```python
from build123d import *

# Parameters (mm, degrees)
SKETCH1_W            = 50.8
SKETCH1_H            = 38.1
SKETCH1_R            = 13.335
BOSS_EXTRUDE2_DEPTH  = 25.4
CUT_EXTRUDE1_REACH   = 42.66
SKETCH2_W            = 25.4
SKETCH2_H            = 2.54
SKETCH3_R            = 2.665
CUT_EXTRUDE2_DEPTH   = 53.363441445
CUT_EXTRUDE3_DEPTH   = 10
CUT_EXTRUDE4_START   = -1.5
CUT_EXTRUDE4_DEPTH   = 1.5
SKETCH6_W            = 50.8
SKETCH6_H            = 38.1
SKETCH6_R            = 6.477
BOSS_EXTRUDE3_DEPTH  = 6.35
BOSS_EXTRUDE4_DEPTH  = 44.45
BOSS_EXTRUDE5_DEPTH  = 6.604
SKETCH11_W           = 57.15
SKETCH11_H           = 127
BOSS_EXTRUDE6_DEPTH  = 10.16
CUT_EXTRUDE6_REACH   = 147.3
SKETCH12_R           = 7.62
SKETCH13_R           = 14.351
CUT_EXTRUDE7_DEPTH   = 7.9375
CUT_EXTRUDE8_REACH   = 147.3
CUT_EXTRUDE11_REACH  = 141.019
CUT_EXTRUDE12_REACH  = 147.3
SKETCH16_W           = 57.15
SKETCH16_H           = 7.545
SKETCH17_W           = 17.78
SKETCH17_H           = 23.9
BOSS_EXTRUDE7_DEPTH  = 3.175
BOSS_EXTRUDE8_DEPTH  = 3.175
BOSS_EXTRUDE10_DEPTH = 3.175
SKETCH20_W           = 17.78
SKETCH20_H           = 23.9
BOSS_EXTRUDE11_DEPTH = 3.175
CUT_EXTRUDE13_REACH  = 129.55
SKETCH21_R           = 2.665


with BuildPart() as part:
    # Sketch1 → Boss-Extrude2 (new body)
    with BuildSketch(Plane(origin=(0, 0, 0), x_dir=(1, 0, 0), z_dir=(0, 1, 0))):
        Rectangle(SKETCH1_W, SKETCH1_H)
        with Locations(Location((0, 0, 0), (0, 0, 270))):
            Circle(SKETCH1_R, mode=Mode.SUBTRACT)
    extrude(amount=BOSS_EXTRUDE2_DEPTH)

    # Sketch2 → Cut-Extrude1 (cut, up to next)
    with BuildSketch(Plane(origin=(0, 25.4, 0), x_dir=(1, 0, 0), z_dir=(0, 1, 0)), mode=Mode.PRIVATE) as cut_extrude1_sk1:
        with Locations((12.7, 0)):
            Rectangle(SKETCH2_W, SKETCH2_H)
    cut_extrude1_tool1 = extrude(cut_extrude1_sk1.sketch, amount=-CUT_EXTRUDE1_REACH, mode=Mode.PRIVATE) & part.part
    add(cut_extrude1_tool1.solids().sort_by_distance((12.7, 25.4, 0))[0], mode=Mode.SUBTRACT)

    # Sketch3 → Cut-Extrude2 (cut, through all)
    with BuildSketch(Plane.XY.offset(19.05)):
        with Locations((19.05, 19.05)):
            Circle(SKETCH3_R)
        with Locations((19.05, 6.35)):
            Circle(SKETCH3_R)
    extrude(amount=-CUT_EXTRUDE2_DEPTH, mode=Mode.SUBTRACT)

    # Sketch4 → Cut-Extrude3 (cut)
    with BuildSketch(Plane(origin=(0, 0, -19.05), x_dir=(-1, 0, 0), z_dir=(0, 0, -1))):
        Polygon((-19.05, 24.823502692), (-24.05, 21.936751346), (-24.05, 16.163248654), (-19.05, 13.276497308), (-14.05, 16.163248654), (-14.05, 21.936751346), align=None)
        Polygon((-19.05, 12.123502692), (-24.05, 9.236751346), (-24.05, 3.463248654), (-19.05, 0.576497308), (-14.05, 3.463248654), (-14.05, 9.236751346), align=None)
    extrude(amount=-CUT_EXTRUDE3_DEPTH, mode=Mode.SUBTRACT)

    # Sketch5 → Cut-Extrude4 (cut)
    with BuildSketch(Plane(origin=(0, 25.4, 0), x_dir=(1, 0, 0), z_dir=(0, 1, 0)).offset(CUT_EXTRUDE4_START)):
        with BuildLine():
            Line((-19.05, -19.05), (-9.429268927, -9.429268927))
            ThreePointArc((-9.429268927, -9.429268927), (4.509949975, -12.549206199), (13.27438605, -1.27))
            Line((13.27438605, -1.27), (25.4, -1.27))
            Line((25.4, -1.27), (25.4, -19.05))
            Line((25.4, -19.05), (-19.05, -19.05))
        make_face()
    extrude(amount=CUT_EXTRUDE4_DEPTH, mode=Mode.SUBTRACT)

    # Sketch6 → Boss-Extrude3 (add)
    with BuildSketch(Plane(origin=(0, 25.4, 0), x_dir=(1, 0, 0), z_dir=(0, 1, 0))):
        Rectangle(SKETCH6_W, SKETCH6_H)
        with Locations(Location((0, 0, 0), (0, 0, 270))):
            Circle(SKETCH6_R, mode=Mode.SUBTRACT)
    extrude(amount=BOSS_EXTRUDE3_DEPTH)

    # Sketch8 → Boss-Extrude4 (add)
    with BuildSketch(Plane(origin=(0, 31.75, 0), x_dir=(1, 0, 0), z_dir=(0, 1, 0))):
        with BuildLine():
            Line((-25.4, 19.05), (25.4, 19.05))
            Line((25.4, 19.05), (25.4, 0))
            Line((25.4, 0), (6.477, 0))
            ThreePointArc((6.477, 0), (0, 6.477), (-6.477, 0))
            Line((-6.477, 0), (-25.4, 0))
            Line((-25.4, 0), (-25.4, 19.05))
        make_face()
    extrude(amount=BOSS_EXTRUDE4_DEPTH)

    # Sketch10 → Boss-Extrude5 (add)
    with BuildSketch(Plane(origin=(0, 76.2, 0), x_dir=(1, 0, 0), z_dir=(0, 1, 0))):
        with BuildLine():
            Line((-25.4, 19.05), (-25.4, 0))
            Line((-25.4, 0), (-13.97, 0))
            ThreePointArc((-13.97, 0), (0, 13.97), (13.97, 0))
            Line((13.97, 0), (25.4, 0))
            Line((25.4, 0), (25.4, 19.05))
            Line((25.4, 19.05), (-25.4, 19.05))
        make_face()
    extrude(amount=BOSS_EXTRUDE5_DEPTH)

    # Sketch11 → Boss-Extrude6 (add)
    with BuildSketch(Plane(origin=(0, 82.804, 0), x_dir=(1, 0, 0), z_dir=(0, 1, 0))):
        with Locations((0, 44.45)):
            Rectangle(SKETCH11_W, SKETCH11_H)
    extrude(amount=BOSS_EXTRUDE6_DEPTH)

    # Sketch12 → Cut-Extrude6 (cut, up to next)
    with BuildSketch(Plane(origin=(0, 92.964, 0), x_dir=(1, 0, 0), z_dir=(0, 1, 0)), mode=Mode.PRIVATE) as cut_extrude6_sk1:
        with Locations(Location((0, 0, 0), (0, 0, 270))):
            Circle(SKETCH12_R)
    cut_extrude6_tool1 = extrude(cut_extrude6_sk1.sketch, amount=-CUT_EXTRUDE6_REACH, mode=Mode.PRIVATE) & part.part
    add(cut_extrude6_tool1.solids().sort_by_distance((0, 92.964, 0))[0], mode=Mode.SUBTRACT)

    # Sketch13 → Cut-Extrude7 (cut)
    with BuildSketch(Plane(origin=(0, 92.964, 0), x_dir=(1, 0, 0), z_dir=(0, 1, 0))):
        with Locations(Location((0, 0, 0), (0, 0, 270))):
            Circle(SKETCH13_R)
    extrude(amount=-CUT_EXTRUDE7_DEPTH, mode=Mode.SUBTRACT)

    # Sketch14 → Cut-Extrude8 (cut, up to next)
    with BuildSketch(Plane(origin=(0, 92.964, 0), x_dir=(1, 0, 0), z_dir=(0, 1, 0)), mode=Mode.PRIVATE) as cut_extrude8_sk1:
        with BuildLine():
            Line((-19.177, 65.405), (-19.177, 71.755))
            ThreePointArc((-19.177, 71.755), (0, 90.932), (19.177, 71.755))
            Line((19.177, 71.755), (19.177, 65.405))
            ThreePointArc((19.177, 65.405), (0, 46.228), (-19.177, 65.405))
        make_face()
    cut_extrude8_tool1 = extrude(cut_extrude8_sk1.sketch, amount=-CUT_EXTRUDE8_REACH, mode=Mode.PRIVATE) & part.part
    add(cut_extrude8_tool1.solids().sort_by_distance((0, 92.964, -68.58))[0], mode=Mode.SUBTRACT)

    # Sketch15 → Cut-Extrude11 (cut, up to next)
    with BuildSketch(Plane.XZ.offset(-82.804), mode=Mode.PRIVATE) as cut_extrude11_sk1:
        with BuildLine():
            Line((-21.03, -88.975), (-21.03, -95.325))
            ThreePointArc((-21.03, -95.325), (-23.57, -97.865), (-26.11, -95.325))
            Line((-26.11, -95.325), (-26.11, -88.975))
            ThreePointArc((-26.11, -88.975), (-23.57, -86.435), (-21.03, -88.975))
        make_face()
    cut_extrude11_tool1 = extrude(cut_extrude11_sk1.sketch, amount=-CUT_EXTRUDE11_REACH, mode=Mode.PRIVATE) & part.part
    # Sketch15 → Cut-Extrude11 (cut, up to next)
    with BuildSketch(Plane.XZ.offset(-82.804), mode=Mode.PRIVATE) as cut_extrude11_sk2:
        with BuildLine():
            Line((26.11, -88.975), (26.11, -95.325))
            ThreePointArc((26.11, -95.325), (23.57, -97.865), (21.03, -95.325))
            Line((21.03, -95.325), (21.03, -88.975))
            ThreePointArc((21.03, -88.975), (23.57, -86.435), (26.11, -88.975))
        make_face()
    cut_extrude11_tool2 = extrude(cut_extrude11_sk2.sketch, amount=-CUT_EXTRUDE11_REACH, mode=Mode.PRIVATE) & part.part
    # Sketch15 → Cut-Extrude11 (cut, up to next)
    with BuildSketch(Plane.XZ.offset(-82.804), mode=Mode.PRIVATE) as cut_extrude11_sk3:
        with BuildLine():
            Line((26.11, -41.835), (26.11, -48.185))
            ThreePointArc((26.11, -48.185), (23.57, -50.725), (21.03, -48.185))
            Line((21.03, -48.185), (21.03, -41.835))
            ThreePointArc((21.03, -41.835), (23.57, -39.295), (26.11, -41.835))
        make_face()
    cut_extrude11_tool3 = extrude(cut_extrude11_sk3.sketch, amount=-CUT_EXTRUDE11_REACH, mode=Mode.PRIVATE) & part.part
    # Sketch15 → Cut-Extrude11 (cut, up to next)
    with BuildSketch(Plane.XZ.offset(-82.804), mode=Mode.PRIVATE) as cut_extrude11_sk4:
        with BuildLine():
            Line((-21.03, -41.835), (-21.03, -48.185))
            ThreePointArc((-21.03, -48.185), (-23.57, -50.725), (-26.11, -48.185))
            Line((-26.11, -48.185), (-26.11, -41.835))
            ThreePointArc((-26.11, -41.835), (-23.57, -39.295), (-21.03, -41.835))
        make_face()
    cut_extrude11_tool4 = extrude(cut_extrude11_sk4.sketch, amount=-CUT_EXTRUDE11_REACH, mode=Mode.PRIVATE) & part.part
    add(cut_extrude11_tool1.solids().sort_by_distance((-23.57, 82.804, -92.15))[0], mode=Mode.SUBTRACT)
    add(cut_extrude11_tool2.solids().sort_by_distance((23.57, 82.804, -92.15))[0], mode=Mode.SUBTRACT)
    add(cut_extrude11_tool3.solids().sort_by_distance((23.57, 82.804, -45.01))[0], mode=Mode.SUBTRACT)
    add(cut_extrude11_tool4.solids().sort_by_distance((-23.57, 82.804, -45.01))[0], mode=Mode.SUBTRACT)

    # Sketch16 → Cut-Extrude12 (cut, up to next)
    with BuildSketch(Plane(origin=(0, 92.964, 0), x_dir=(1, 0, 0), z_dir=(0, 1, 0)), mode=Mode.PRIVATE) as cut_extrude12_sk1:
        with Locations((0, 104.1775)):
            Rectangle(SKETCH16_W, SKETCH16_H)
    cut_extrude12_tool1 = extrude(cut_extrude12_sk1.sketch, amount=-CUT_EXTRUDE12_REACH, mode=Mode.PRIVATE) & part.part
    add(cut_extrude12_tool1.solids().sort_by_distance((0, 92.964, -104.1775))[0], mode=Mode.SUBTRACT)

    # Sketch17 → Boss-Extrude7 (add)
    with BuildSketch(Plane(origin=(25.4, 0, 0), x_dir=(0, 0, -1), z_dir=(1, 0, 0))):
        with Locations((-10.16, 11.95)):
            Rectangle(SKETCH17_W, SKETCH17_H)
        Polygon((19.05, 0), (19.05, 82.804), (0, 82.804), (0, 31.75), (-19.05, 31.75), (-19.05, 25.4), (1.27, 25.4), (1.27, 0), align=None)
    extrude(amount=BOSS_EXTRUDE7_DEPTH)

    # Sketch18 → Boss-Extrude8 (add)
    with BuildSketch(Plane.ZY.offset(25.4)):
        Polygon((-19.05, 0), (19.05, 0), (19.05, 31.75), (0, 31.75), (0, 82.804), (-19.05, 82.804), align=None)
    extrude(amount=BOSS_EXTRUDE8_DEPTH)

    # Sketch19 → Boss-Extrude10 (add)
    with BuildSketch(Plane.ZY.offset(28.575)):
        Polygon((0, 92.964), (-100.405, 92.964), (-100.405, 82.804), (-19.05, 82.804), (-19.05, 31.75), (0, 31.75), (0, 82.804), (19.05, 82.804), (19.05, 92.964), align=None)
        Polygon((0, 31.75), (-19.05, 31.75), (-19.05, 0), (19.05, 0), (19.05, 31.75), align=None)
        Polygon((-19.05, 82.804), (-100.405, 82.804), (-19.05, 31.75), align=None)
    extrude(amount=BOSS_EXTRUDE10_DEPTH)

    # Sketch20 → Boss-Extrude11 (add)
    with BuildSketch(Plane(origin=(28.575, 0, 0), x_dir=(0, 0, -1), z_dir=(1, 0, 0))):
        Polygon((19.05, 31.75), (100.405, 82.804), (100.405, 92.964), (-19.05, 92.964), (-19.05, 82.804), (0, 82.804), (0, 31.75), (-19.05, 31.75), (-19.05, 25.4), (1.27, 25.4), (1.27, 0), (19.05, 0), align=None)
        with Locations((-10.16, 11.95)):
            Rectangle(SKETCH20_W, SKETCH20_H)
    extrude(amount=BOSS_EXTRUDE11_DEPTH)

    # Sketch21 → Cut-Extrude13 (cut, up to next)
    with BuildSketch(Plane(origin=(0, 0, -19.05), x_dir=(-1, 0, 0), z_dir=(0, 0, -1)), mode=Mode.PRIVATE) as cut_extrude13_sk1:
        with Locations((22.575, 57.15)):
            Circle(SKETCH21_R)
    cut_extrude13_tool1 = extrude(cut_extrude13_sk1.sketch, amount=-CUT_EXTRUDE13_REACH, mode=Mode.PRIVATE) & part.part
    # Sketch21 → Cut-Extrude13 (cut, up to next)
    with BuildSketch(Plane(origin=(0, 0, -19.05), x_dir=(-1, 0, 0), z_dir=(0, 0, -1)), mode=Mode.PRIVATE) as cut_extrude13_sk2:
        with Locations((-22.575, 57.15)):
            Circle(SKETCH21_R)
    cut_extrude13_tool2 = extrude(cut_extrude13_sk2.sketch, amount=-CUT_EXTRUDE13_REACH, mode=Mode.PRIVATE) & part.part
    add(cut_extrude13_tool1.solids().sort_by_distance((-22.575, 57.15, -19.05))[0], mode=Mode.SUBTRACT)
    add(cut_extrude13_tool2.solids().sort_by_distance((22.575, 57.15, -19.05))[0], mode=Mode.SUBTRACT)


solid = part.part
```
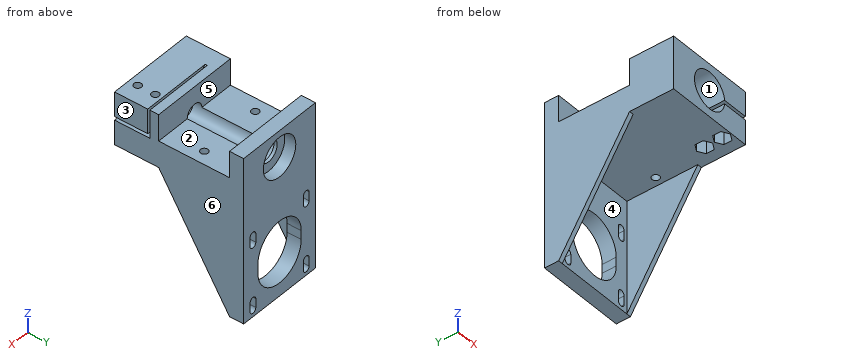
The model under review builds one solid part; all positions refer to its coordinate system, in mm. Face numbers are marked on the shaded views. A direction names the side the tool comes from. Round coordinates to 2 decimals unless told otherwise and drop trailing zeros. Order: outer loops, then holes, each group sorted by start corner. A loop starts at its lowest first (then second) coordinate and runs counter-clockwise, first axis right, second up.
(1) Take a section at D-D, the plane z = -61.5. State the section outline as (x, y) points (3 decimals).
Working result:
outline: (-31.75, 58.389) - (-28.575, 58.389) - (-28.575, 82.804) - (-18.775, 82.804) - (-18.775, 92.964) - (-31.75, 92.964) - close; (18.775, 82.804) - (28.575, 82.804) - (28.575, 58.389) - (31.75, 58.389) - (31.75, 92.964) - (18.775, 92.964) - close
(2) Take a section at B-B, the plane z = 5. Count the separate pieces of the cut face and the enclosed holes in it, plus the area to 3 significant figures.
Working result:
separate pieces: 5
enclosed holes: 2
area: 1,670 mm2
(3) Take a section at C-C, the plane x = -23.57. State the section outline as (y, z) points (3 decimals).
Working result:
outline: (0, -19.05) - (54.678, -19.05) - (54.678, 0) - (31.75, 0) - (31.75, 19.05) - (0, 19.05) - close; (59.622, -19.05) - (82.804, -19.05) - (82.804, -39.295) - (92.964, -39.295) - (92.964, 19.05) - (82.804, 19.05) - (82.804, 0) - (59.622, 0) - close; (82.804, -100.405) - (92.964, -100.405) - (92.964, -97.865) - (82.804, -97.865) - close; (82.804, -86.435) - (92.964, -86.435) - (92.964, -50.725) - (82.804, -50.725) - close
(4) Tool access review of the marked faces 4, 5 and 6: name each direction out of +Z, -Z, +X, -X, +Y, -Y from which nothing blocks a thin tool from reaching the whole face with its end or side.
Working result:
face 4: -Z, -Y
face 5: +Z, +X, -X
face 6: +Z, -Z, +X, +Y, -Y
(5) For P1, Ø6, axis at x = -22.5, y = 13.5, coming from the -Z side; P2, Ø4.5, axis at x = 19.05, y = 19.05, coming from the -Z side; P3, Ø6, axis at x = 19.5, y = 38.5, coming from the +Z side; P4, Ø4, axis at x = 3.5, z = -6, coming from the +Y side, all flat-tipped, find the tip position at first contact; note any pin that passes through.
Working result:
P1: stops at z = -19.05
P2: passes through
P3: stops at z = 0
P4: stops at y = 85.03
(6) Take a section at A-A, the plane y = 6.35. State the section outline as (x, z) points (3 decimals), plus the area to 3 significant figures.
Working result:
outline: (-31.75, -19.05) - (14.05, -19.05) - (14.05, -9.05) - (16.385, -9.05) - (16.385, -1.27) - (13.274, -1.27) arc R13.335 cw (long way) to (13.274, 1.27) - (16.385, 1.27) - (16.385, 19.05) - (-31.75, 19.05) - close; (21.715, -9.05) - (24.05, -9.05) - (24.05, -19.05) - (31.75, -19.05) - (31.75, -1.27) - (21.715, -1.27) - close; (21.715, 1.27) - (31.75, 1.27) - (31.75, 19.05) - (21.715, 19.05) - close
area: 1,580 mm2
(7) Wall thickness on L1, parallel to X at y = 54, z = -48 (3 decimals); L2, parallel to X at y = 57, z = -11; L3, parallel to Z at x = 1, y = 87 (3 decimals): over which ranges is each line inside the solid? List them lowest first.
Working result:
L1: x = -31.75 to -28.575, 28.575 to 31.75
L2: x = -31.75 to -25.24, -19.91 to 19.91, 25.24 to 31.75
L3: z = -100.405 to -90.906, -46.254 to -14.316, 14.316 to 19.05
(8) Mouldability with a two-part tool opening along X and no side actions: class the marked faces 1, 2 and 3 as released by +X, released by -X, zero draft, split by the parting line, or undercut.
Working result:
face 1: undercut
face 2: zero draft
face 3: released by +X
